For this review, take the finished solid that the model builds, in its own axes (mm). Face numbers are marked on the shaded views. Coordinates: 2 decimals unless noted, no trailing zeros. Write each loop counter-clockwise with the first axis right and the second up, starting at its lowest first coordinate (ties: lowest second). Pieces come first, ordered by that corner, then holes.
```python
from build123d import *

# Parameters (mm, degrees)
BOSS_EXTRUDE1_DEPTH = 10.16
SKETCH2_W           = 11.43
SKETCH2_H           = 11.43
SKETCH2_R           = 2
BOSS_EXTRUDE2_DEPTH = 2.54
FILLET2_R           = 0.762


with BuildPart() as part:
    # Sketch1 → Boss-Extrude1 (new body)
    with BuildSketch(Plane(origin=(0, 0, 0), x_dir=(1, 0, 0), z_dir=(0, 1, 0))):
        Polygon((0, 0), (0, 16.764), (-3.81, 16.764), (-3.81, 3.81), (-16.764, 3.81), (-16.764, 0), align=None)
    extrude(amount=BOSS_EXTRUDE1_DEPTH)

    # Sketch2 → Boss-Extrude2 (add)
    with BuildSketch(Plane(origin=(0, 0, 0), x_dir=(1, 0, 0), z_dir=(0, 1, 0))):
        with Locations((-5.715, 5.715)):
            Rectangle(SKETCH2_W, SKETCH2_H)
        with Locations(Location((-7.874, 7.874, 0), (0, 0, 270))):
            Circle(SKETCH2_R, mode=Mode.SUBTRACT)
    extrude(amount=BOSS_EXTRUDE2_DEPTH)

    # Sketch3 → section 1 of loft3
    with BuildSketch(Plane(origin=(0, 15.24, 0), x_dir=(1, 0, 0), z_dir=(0, 1, 0)), mode=Mode.PRIVATE) as loft3_s1:
        with BuildLine():
            Line((-3.2004, 3.175), (-3.2004, 16.764))
            Line((-3.2004, 16.764), (-3.81, 16.764))
            Line((-3.81, 16.764), (-3.81, 3.81))
            Line((-3.81, 3.81), (-16.764, 3.81))
            Line((-16.764, 3.81), (-16.764, 3.175))
            Line((-16.764, 3.175), (-3.2004, 3.175))
        make_face()
    # loft from a face of the part (loft3)
    loft([part.faces().sort_by_distance((-0.237078762, 10.16, -8.382))[0], loft3_s1.sketch])

    # Mirror4: part across plane


with BuildPart() as part_1:
    add(part.part)
    add(part.part.mirror(Plane(origin=(0, 10.16, -16.764), x_dir=(1, 0, 0), z_dir=(0, 0, 1))))

    # Fillet2
    # the kernel refuses this fillet: 0.762 mm, written as the material it takes off along each edge
    with BuildSketch(Plane(origin=(-16.764, -1.905, -3.81), x_dir=(0, 0, 1), z_dir=(0, 1, 0)), Plane(origin=(-16.764, -1.905, -29.718), x_dir=(1, 0, 0), z_dir=(0, 1, 0))) as fillet2_piece_1:
        with BuildLine():
            CenterArc((FILLET2_R, FILLET2_R), FILLET2_R, 180, 90)
            Line((0, FILLET2_R), (0, 0))
            Line((0, 0), (FILLET2_R, 0))
        make_face()
    extrude(amount=19.05, mode=Mode.SUBTRACT)
    with BuildSketch(Plane(origin=(-11.43, -1.905, -11.43), x_dir=(0, 0, 1), z_dir=(0, 1, 0))) as fillet2_piece_2:
        with BuildLine():
            CenterArc((FILLET2_R, FILLET2_R), FILLET2_R, 180, 90)
            Line((0, FILLET2_R), (0, 0))
            Line((0, 0), (FILLET2_R, 0))
        make_face()
    extrude(amount=6.35, mode=Mode.SUBTRACT)
    with BuildSketch(Plane(origin=(-17.819841757, 15.24, -3.175), x_dir=(0, 0, -1), z_dir=(1, 0, 0)), Plane(origin=(-17.819841757, 15.24, -30.353), x_dir=(0, -0.8479983040050892, -0.5299989400031782), z_dir=(1, 0, 0))) as fillet2_piece_3:
        with BuildLine():
            CenterArc((FILLET2_R * 0.554247641507, -FILLET2_R), FILLET2_R, 90, 57.994616792)
            Line((-FILLET2_R * 0.293750662498, -FILLET2_R * 0.470001059997), (0, 0))
            Line((0, 0), (FILLET2_R * 0.554247641507, 0))
        make_face()
    extrude(amount=15.675283514, mode=Mode.SUBTRACT)
    with BuildSketch(Plane(origin=(-3.2004, 15.24, -31.404379485), x_dir=(-1, 0, 0), z_dir=(0, 0, 1))) as fillet2_piece_4:
        with BuildLine():
            CenterArc((FILLET2_R * 0.551905241549, FILLET2_R), FILLET2_R, 212.210927724, 57.789072276)
            Line((-FILLET2_R * 0.29418627649, FILLET2_R * 0.466962343635), (0, 0))
            Line((0, 0), (FILLET2_R * 0.551905241549, 0))
        make_face()
    extrude(amount=29.28075897, mode=Mode.SUBTRACT)
    with BuildSketch(Plane(origin=(-16.764, 8.544563231, 1.009647981), x_dir=(1, 0, 0), z_dir=(0, 0.847998304005088, -0.5299989400031799))) as fillet2_piece_5:
        with BuildLine():
            CenterArc((FILLET2_R, FILLET2_R), FILLET2_R, 180, 90)
            Line((0, FILLET2_R), (0, 0))
            Line((0, 0), (FILLET2_R, 0))
        make_face()
    extrude(amount=9.800578019, mode=Mode.SUBTRACT)
    with BuildSketch(Plane(origin=(-17.310346811, 10.16, 0), x_dir=(0, 0.8479983040050875, -0.5299989400031807), z_dir=(1, 0, 0)), Plane(origin=(-17.310346811, 10.16, -33.528), x_dir=(0, -1, 0), z_dir=(1, 0, 0))) as fillet2_piece_6:
        with BuildLine():
            CenterArc((FILLET2_R * 0.286796226411, -FILLET2_R), FILLET2_R, 90, 32.005383208)
            Line((-FILLET2_R * 0.243202713592, -FILLET2_R * 0.152001695995), (0, 0))
            Line((0, 0), (FILLET2_R * 0.286796226411, 0))
        make_face()
    extrude(amount=17.856693623, mode=Mode.SUBTRACT)
    with BuildSketch(Plane(origin=(-11.43, -1.905, -22.098), x_dir=(0, 0, -1), z_dir=(0, 1, 0))) as fillet2_piece_7:
        with BuildLine():
            CenterArc((FILLET2_R, -FILLET2_R), FILLET2_R, 90, 90)
            Line((0, -FILLET2_R), (0, 0))
            Line((0, 0), (FILLET2_R, 0))
        make_face()
    extrude(amount=6.35, mode=Mode.SUBTRACT)
    with BuildSketch(Plane(origin=(-16.764, 8.544563231, -34.537647981), x_dir=(1, 0, 0), z_dir=(0, 0.847998304005088, 0.5299989400031797))) as fillet2_piece_8:
        with BuildLine():
            CenterArc((FILLET2_R, -FILLET2_R), FILLET2_R, 90, 90)
            Line((0, -FILLET2_R), (0, 0))
            Line((0, 0), (FILLET2_R, 0))
        make_face()
    extrude(amount=9.800578019, mode=Mode.SUBTRACT)
    with BuildSketch(Plane(origin=(0, 10.16, -34.078046802), x_dir=(0, -1, 0), z_dir=(0, 0, 1))) as fillet2_piece_9:
        with BuildLine():
            CenterArc((FILLET2_R * 0.288738478649, -FILLET2_R), FILLET2_R, 90, 32.210927724)
            Line((-FILLET2_R * 0.244299177716, -FILLET2_R * 0.153908481961), (0, 0))
            Line((0, 0), (FILLET2_R * 0.288738478649, 0))
        make_face()
    extrude(amount=34.628093604, mode=Mode.SUBTRACT)


solid = part_1.part
```
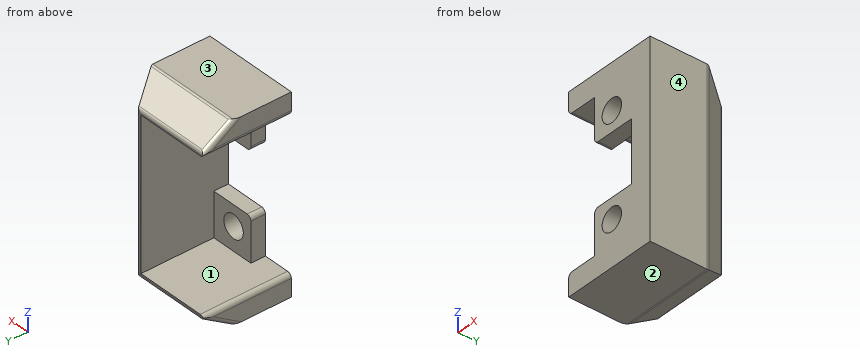
1) Consider section B-B (z = -20.5). Give the boundary of the cut face in (x, y), then the cut area to 3 significant figures.
2) Consider section D-D (x = -7.25). Count the separate pieces of the cut face and the enclosed holes in it, then the cut area to 3 significant figures.
3) For L1, parallel to Z at x = -16, y = 4; L2, parallel to Z at x = -7.25, y = 2; L3, parallel to Z at x = -8.75, y = 2, list the stretches that pass through material, from the lowest coordinate up.
4) Clearance check with flat-ended pins moving along their axes: P1, Ø3, axis at y = 2, z = -6.5, coming from the -X side; P2, Ø1.5, axis at y = 12.5, z = -18.5, coming from the -X side; P3, Ø4, axis at x = -9, z = -25, coming from the +Y side. State where each tip first meets the part, or that it passes through.
5) The part is to be moulded in two halves that separate along Z. For the marked faces 1, 2, 3 and 4, say which applies: pulls with the +Z half, pulls with the -Z half, needs draft (parallel to the pull), parting line crosses it, or undercut.
6) Consider section A-A (y = 4.25). Give the boundary of the cut face in (x, z), then the cut area to 3 significant figures.
7) Consider section C-C (z = -24). Give the boundary of the cut face in (x, y), then the cut area to 3 significant figures.
Results:
1. outline: (-3.81, 0) - (0, 0) - (0, 9.94) arc R0.76 ccw to (-0.12, 10.35) - (-2.98, 14.88) arc R0.76 ccw to (-3.62, 15.24) - (-3.81, 15.24) - close
1. area: 49.9 mm2
2. separate pieces: 4
2. enclosed holes: 0
2. area: 119 mm2
3. L1: z = -33.53 to -29.72, -3.81 to 0
3. L2: z = -33.53 to -27.55, -23.75 to -22.1, -11.43 to -9.77, -5.97 to 0
3. L3: z = -33.53 to -27.45, -23.86 to -22.1, -11.43 to -9.67, -6.08 to 0
4. P1: stops at x = -11.43
4. P2: stops at x = -3.81
4. P3: stops at y = 2.54
5. face 1: undercut
5. face 2: pulls with the -Z half
5. face 3: pulls with the +Z half
5. face 4: needs draft
6. outline: (-16.76, -33.53) - (0, -33.53) - (0, 0) - (-16.76, 0) - (-16.76, -3.05) arc R0.76 ccw to (-16, -3.81) - (-3.81, -3.81) - (-3.81, -29.72) - (-16, -29.72) arc R0.76 ccw to (-16.76, -30.48) - close
6. area: 226 mm2
7. outline: (-11.43, 0) - (-9, 0) - (-9, 2.54) - (-11.43, 2.54) - close; (-6.75, 0) - (0, 0) - (0, 9.94) arc R0.76 ccw to (-0.12, 10.35) - (-2.98, 14.88) arc R0.76 ccw to (-3.62, 15.24) - (-3.81, 15.24) - (-3.81, 2.54) - (-6.75, 2.54) - close
7. area: 63.5 mm2
